from build123d import *

# Parameters (mm, degrees)
SKETCH1_W           = 60
SKETCH1_H           = 60
BOSS_EXTRUDE1_DEPTH = 47
FILLET1_R           = 5
SKETCH2_R           = 27
BOSS_EXTRUDE2_DEPTH = 60
SKETCH3_R           = 5
BOSS_EXTRUDE3_DEPTH = 30


with BuildPart() as part:
    # Sketch1 → Boss-Extrude1 (new body)
    with BuildSketch(Plane(origin=(0, 0, 0), x_dir=(1, 0, 0), z_dir=(0, 1, 0))):
        Rectangle(SKETCH1_W, SKETCH1_H)
    extrude(amount=BOSS_EXTRUDE1_DEPTH)

    # Fillet1
    fillet1_edges = [part.edges().sort_by_distance(p)[0] for p in [
        (30, 23.5, 30),
        (-30, 23.5, 30),
        (-30, 23.5, -30),
        (30, 23.5, -30),
    ]]
    fillet(fillet1_edges, radius=FILLET1_R)

    # Sketch2 → Boss-Extrude2 (add)
    with BuildSketch(Plane(origin=(0, 47, 0), x_dir=(1, 0, 0), z_dir=(0, 1, 0))):
        Circle(SKETCH2_R)
    extrude(amount=BOSS_EXTRUDE2_DEPTH)

    # Sketch3 → Boss-Extrude3 (add)
    with BuildSketch(Plane.XZ):
        with Locations((0, 10)):
            Circle(SKETCH3_R)
    extrude(amount=BOSS_EXTRUDE3_DEPTH)


solid = part.part
For this review, take the finished solid that the model builds, in its own axes (mm). A direction names the side the tool comes from. Coordinates: 2 decimals unless noted, no trailing zeros. Loops run counter-clockwise (first coordinate to the right, second up) from the corner with the lowest first, then second, coordinate; pieces in that order, holes last. Notation, with made-up numbers: (56, 38) - (93, 38) arc R18 cw to (93, 61) - close; hole circle Ø6 at (-5.5, 27.25). An arc over 180 degrees is marked (long way). Use a Markdown table: item, result. Add a question column.
Item 1: We need section B-B (x = 0). Give the boundary of the cut face in (y, z), and give its area (3 significant figures).
Item 2: We need section D-D (z = 11.5). Give the boundary of the cut face in (x, y).
Item 3: Tool access review of faces 1 (the face through (-27, 47, -7)), 2 (the face through (0, 107, 0)): name each direction out of +Z, -Z, +X, -X, +Y, -Y from which nothing blocks a thin tool from reaching the whole face with its end or side.
Item 4: Mouldability with a two-part tool opening along Z and no side actions: class faces 3 (the face through (28, 24, 29)), 4 (the face through (-29, 24, -28)), 5 (the face through (-0.651, -14.79, 14.957)), 6 (the face through (30, 23, 0)) as pulls with the +Z half, pulls with the -Z half, needs draft (parallel to the pull), parting line crosses it, or undercut.
Item 5: Insertion check: pin 1 Ø12 at (x, z) = (-17, -7) entering from -Y; pin 2 Ø1.5 at (x, y) = (-12, 50.5) entering from +Z; pin 3 Ø2 at (y, z) = (65.5, -20) entering from +X. Each pin has a flat end and moves straight along its axis. Give the tip position at first contact, or say it passes through.
Item 6: For line 1 (Y direction, x = -19, z = 12); line 2 (Y direction, x = 27, z = 11); line 3 (X direction, y = 79, z = 14), list the stretches that pass through material, from the lowest coordinate up.
Item 7: We need section C-C (y = 81). Give the boundary of the cut face in (x, z).
Item 8: We need section A-A (z = 0). Give the boundary of the cut face in (x, y), and give its area (3 significant figures).
Results list:
| question | item | result |
|---|---|---|
| 1 | outline | (-30, 5) - (0, 5) - (0, -30) - (47, -30) - (47, -27) - (107, -27) - (107, 27) - (47, 27) - (47, 30) - (0, 30) - (0, 15) - (-30, 15) - close |
| 1 | area | 6,360 mm^2 |
| 2 | outline | (-30, 0) - (-4.77, 0) - (-4.77, -30) - (4.77, -30) - (4.77, 0) - (30, 0) - (30, 47) - (24.43, 47) - (24.43, 107) - (-24.43, 107) - (-24.43, 47) - (-30, 47) - close |
| 3 | face 1 | +Y |
| 3 | face 2 | +Z, -Z, +X, -X, +Y |
| 4 | face 3 | pulls with the +Z half |
| 4 | face 4 | pulls with the -Z half |
| 4 | face 5 | parting line crosses it |
| 4 | face 6 | needs draft |
| 5 | pin 1 | stops at y = 0 |
| 5 | pin 2 | stops at z = 24.54 |
| 5 | pin 3 | stops at x = 19.18 |
| 6 | line 1 | y = 0 to 107 |
| 6 | line 2 | y = 0 to 47 |
| 6 | line 3 | x = -23.09 to 23.09 |
| 7 | outline | circle Ø54 at (0, 0) |
| 8 | outline | (-30, 0) - (30, 0) - (30, 47) - (27, 47) - (27, 107) - (-27, 107) - (-27, 47) - (-30, 47) - close |
| 8 | area | 6,060 mm^2 |
